Design review of the part built by this model. Coordinates are the model's own, in mm. A direction names the side the tool comes from. Give positions to 0.01 mm unless a question says otherwise; leave off trailing zeros. Write each loop counter-clockwise with the first axis right and the second up, starting at its lowest first coordinate (ties: lowest second). Pieces come first, ordered by that corner, then holes. Notation, with made-up numbers: (0, -31.75) -> (19, -31.75) arc R27 cw to (19, 0.25) -> close; hole circle Ø9 at (-23, 1). An arc over 180 degrees is marked (long way). Answer as a JSON object with one key per item and string values.
Autodesk Inventor part; units mm, degrees
ref_plane "YZ Plane" through (0, 0, 0) normal (1, 0, 0) x (0, 1, 0)
ref_plane "XZ Plane" through (0, 0, 0) normal (0, 1, 0) x (-1, 0, 0)
ref_plane "XY Plane" through (0, 0, 0) normal (0, 0, 1) x (1, 0, 0)
sketch "草圖1" plane through (0, 0, 0) normal (0, 1, 0) x (-1, 0, 0)
  line L0 (-100, 0) -> (-100, -180)
  line L1 (-80, -200) -> (-20, -200)
  line L2 (0, -180) -> (0, 0)
  arc A0 (0, 0) -> (-100, 0) centre (-50, 0) ccw
  arc A1 (-20, -200) -> (0, -180) centre (-20, -180) ccw
  arc A2 (-100, -180) -> (-80, -200) centre (-80, -180) ccw
  line L3 (-50, -180) -> (-50, -20) construction
  line L4 (-46.5, -180) -> (-46.5, -20)
  line L5 (-53.5, -20) -> (-53.5, -180)
  arc A3 (-53.5, -180) -> (-46.5, -180) centre (-50, -180) ccw
  arc A4 (-46.5, -20) -> (-53.5, -20) centre (-50, -20) ccw
  line L6 (-50, -180) -> (110, -180) construction
  line L7 (0, 0) -> (-100, 0) construction
  line L8 (-50, 0) -> (-50, 50) construction
  circle A5 centre (-50, 25) radius 14.5
  point P0 (-50, -100)
  dimension "d5" = 20
  dimension "d6" = 160
  dimension "d7" = 90
  dimension "d8" = 7
  dimension "d12" = 29
sketch "草圖2" plane through (0, 0, 0) normal (0, 1, 0) x (-1, 0, 0)
  line L0 (0, 0) -> (-100, 0)
  line L1 (-50, 0) -> (-50, 50) construction
  circle A0 centre (-50, 25) radius 14.5
  dimension "d9" = 100
  dimension "d10" = 50
  dimension "d11" = 29
extrude "擠出1" add sketch "草圖1" along normal blind 6
(1) For line 1 along Z through (x, y) = (50, 2.6); line 2 along X through (y, z) = (2.05, -128); line 3 along Z through (x, y) = (49, 5.05), list the stretches that pass through material, from the lowest coordinate up.
Here are the results:
{"line 1": "z = -200 to -183.5, -16.5 to 10.5, 39.5 to 50", "line 2": "x = 0 to 46.5, 53.5 to 100", "line 3": "z = -200 to -183.35, -16.65 to 10.53, 39.47 to 49.99"}
(2) The part is to be moulded in two halves that separate along Z. For faces 1 (the cylindrical face through (51.099, 2.958, 49.988)), 2 (the cylindrical face through (5.703, 2.958, -193.986)), 3 (the cylindrical face through (50.1, 3, -16.5)), say which applies: +Z half, -Z half, draft (parallel to the pull), parting line (faces both ways), or undercut.
Here are the results:
{"face 1": "+Z half", "face 2": "-Z half", "face 3": "undercut"}
(3) We need section A-A, the plane x = 50. State the section outline as (y, z) points, then the cut area to 3 significant figures.
Here are the results:
{"outline": "(0, -200) -> (6, -200) -> (6, -183.5) -> (0, -183.5) -> close; (0, -16.5) -> (6, -16.5) -> (6, 10.5) -> (0, 10.5) -> close; (0, 39.5) -> (6, 39.5) -> (6, 50) -> (0, 50) -> close", "area": "324 mm²"}
(4) We need section B-B, the plane z = -88. State the section outline as (x, y) points.
Here are the results:
{"outline": "(0, 0) -> (46.5, 0) -> (46.5, 6) -> (0, 6) -> close; (53.5, 0) -> (100, 0) -> (100, 6) -> (53.5, 6) -> close"}
(5) For faces 4 (the flat face through (100, 3, -89)), 5 (the flat face through (53.5, 3, -99)), list the 3-axis set-ups (+Z, -Z, +X, -X, +Y, -Y) from which the entire face can be reached by the end or side of a thin tool; tool diameter is ignored.
Here are the results:
{"face 4": "+Z, -Z, +X, +Y, -Y", "face 5": "+Y, -Y"}
(6) We need section D-D, the plane z = 16. State the section outline as (x, y) points, then the cut area to 3 significant figures.
Here are the results:
{"outline": "(2.63, 0) -> (38.63, 0) -> (38.63, 6) -> (2.63, 6) -> close; (61.37, 0) -> (97.37, 0) -> (97.37, 6) -> (61.37, 6) -> close", "area": "432 mm²"}
(7) Clearance check with a flat-ended pin moving along its axis: pin 1 (3 mm diameter, centred on x = 14, y = 0.5, fed in from -Z). State where the tip first meets the part, or that it passes through.
Here are the results:
{"pin 1": "stops at z = -199.49"}
(8) We need section C-C, the plane y = 2.65. State the section outline as (x, z) points, then the cut area to 3 significant figures.
Here are the results:
{"outline": "(0, -180) arc R20 ccw to (20, -200) -> (80, -200) arc R20 ccw to (100, -180) -> (100, 0) arc R50 ccw to (0, 0) -> close; hole circle Ø29 at (50, 25); hole (46.5, -180) arc R3.5 ccw to (53.5, -180) -> (53.5, -20) arc R3.5 ccw to (46.5, -20) -> close", "area": "21,900 mm²"}
